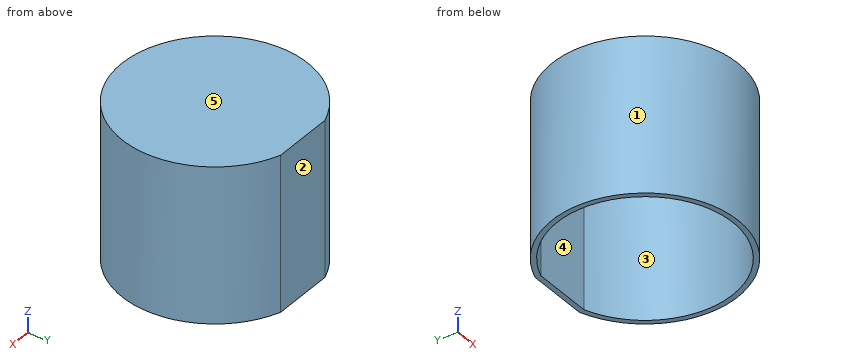
Autodesk Inventor part; units mm, degrees
ref_plane "XZ Plane" through (0, 0, 0) normal (0, 1, 0) x (-1, 0, 0)
ref_plane "XY Plane" through (0, 0, 0) normal (0, 0, 1) x (1, 0, 0)
sketch "Skizze1" plane through (0, 0, 0) normal (0, 0, 1) x (1, 0, 0)
  arc A0 (-29.5804, 85) -> (29.5804, 85) centre (0, 0) ccw
  line L0 (0, 120) -> (0, -125)
  line L1 (-126, 0) -> (126, 0)
  line L2 (-29.5804, 85) -> (29.5804, 85)
  dimension "d0" = 180
  dimension "d1" = 85
extrude "Extrusion1" add sketch "Skizze1" along normal blind 150
shell "Wandstärke1" thickness 5 removed faces 1 at (-9.8601, -16.0312, 0)
ref_plane "Arbeitsebene1" through (0, 0, 0) normal (1, 0, 0) x (0, 1, 0)
properties part number "Testmasse"
Design review of the part built by this model. Coordinates are the model's own, in mm. Face numbers are marked on the shaded views. A direction names the side the tool comes from. Give positions to 0.01 mm unless a question says otherwise; leave off trailing zeros. Write each loop counter-clockwise with the first axis right and the second up, starting at its lowest first coordinate (ties: lowest second). Pieces come first, ordered by that corner, then holes. Notation, with made-up numbers: (82, -21) - (102, -21) arc R23 ccw to (102, 11) - close; hole circle Ø9 at (-26, 56). An arc over 180 degrees is marked (long way). Return JSON: item names as keys, results as strings. Group by question number.
(1) We need section C-C, the plane z = 67. Give the boundary of the cut face in (x, y), then the cut area to 3 significant figures.
(2) We need section B-B, the plane y = 0. Give the boundary of the cut face in (x, z), then the cut area to 3 significant figures.
(3) Mouldability with a two-part tool opening along X and no side actions: class the marked faces 1, 2 and 3 as +X half, -X half, draft (parallel to the pull), parting line (faces both ways), or undercut.
(4) We need section A-A, the plane x = 0. Give the boundary of the cut face in (y, z), then the cut area to 4 significant figures.
(5) To check wall thickness, follow probe 1 along X at (y, z) = (3, 107.5); probe 2 along Y at (x, z) = (0, 106); probe 3 along X at (y, z) = (0, 80). State the ranges of each line that lie inside material, in increasing order.
(6) Insertion check: pin 1 (8 mm diameter, centred on x = -1, y = -57.5, fed in from -Z); pin 2 (8 mm diameter, centred on x = -31.5, z = 71.5, fed in from -Y); pin 3 (3 mm diameter, centred on x = -54.5, z = 127, fed in from -Y). Each pin has a flat end and moves straight along its axis. Give the tip position at first contact, or say it passes through.
(7) Machinability: for the marked faces 4 and 5, which of the approach directions +Z, -Z, +X, -X, +Y, -Y give a long, thin tool a straight path to every point of the face, cutting with its end or side? Answer none if there is none.
Reported:
{
 "1": {"outline": "(-29.58, 85) arc R90 ccw (long way) to (29.58, 85) - close; hole (-28.72, 80) arc R85 ccw (long way) to (28.72, 80) - close", "area": "2,740 mm2"},
 "2": {"outline": "(-90, 0) - (-85, 0) - (-85, 145) - (85, 145) - (85, 0) - (90, 0) - (90, 150) - (-90, 150) - close", "area": "2,350 mm2"},
 "3": {"face 1": "parting line", "face 2": "draft", "face 3": "undercut"},
 "4": {"outline": "(-90, 0) - (-85, 0) - (-85, 145) - (80, 145) - (80, 0) - (85, 0) - (85, 150) - (-90, 150) - close", "area": "2,325 mm2"},
 "5": {"probe 1": "x = -89.95 to -84.95, 84.95 to 89.95", "probe 2": "y = -90 to -85, 80 to 85", "probe 3": "x = -90 to -85, 85 to 90"},
 "6": {"pin 1": "stops at z = 145", "pin 2": "stops at y = -85.7", "pin 3": "stops at y = -72.74"},
 "7": {"face 4": "-Z", "face 5": "+Z, +X, -X, +Y, -Y"}
}
